Autodesk Inventor part; units mm, degrees
ref_plane "Work Plane2" through (0, 5.93, 0) normal (0, 1, 0) x (1, 0, 0)
ref_plane "YZ Plane" through (0, 0, 0) normal (1, 0, 0) x (0, 1, 0)
ref_plane "XZ Plane" through (0, 0, 0) normal (0, 1, 0) x (-1, 0, 0)
ref_plane "Work Plane2" through (0, 5.93, 0) normal (0, 1, 0) x (1, 0, 0)
sketch "Sketch7" plane through (0, 5.93, 0) normal (0, 1, 0) x (1, 0, 0)
  line L0 (-68.89, 72.25) -> (-68.89, 75.38)
  line L1 (-70.59, 75.38) -> (-68.89, 75.38)
  line L2 (-70.59, 83.0068) -> (-70.59, 75.38)
  line L3 (-64.9127, 88.12) -> (-70.59, 83.0068)
  line L4 (-5, 88.12) -> (-64.9127, 88.12)
  arc A0 (1.7, 81.42) -> (-5, 88.12) centre (-5, 81.42) ccw
  line L5 (1.7, 5) -> (1.7, 81.42)
  arc A1 (-5, -1.7) -> (1.7, 5) centre (-5, 5) ccw
  line L6 (-64.9127, -1.7) -> (-5, -1.7)
  line L7 (-70.59, 3.4132) -> (-64.9127, -1.7)
  line L8 (-70.59, 14.5) -> (-70.59, 3.4132)
  line L9 (-68.89, 14.5) -> (-70.59, 14.5)
  line L10 (-68.89, 14.5) -> (-68.89, 17.63)
  line L11 (-70.59, 17.63) -> (-68.89, 17.63)
  line L12 (-70.59, 47.6) -> (-70.59, 17.63)
  line L13 (-68.89, 47.6) -> (-70.59, 47.6)
  line L14 (-68.89, 47.6) -> (-68.89, 50.73)
  line L15 (-70.59, 50.73) -> (-68.89, 50.73)
  line L16 (-70.59, 72.25) -> (-70.59, 50.73)
  line L17 (-68.89, 72.25) -> (-70.59, 72.25)
  line L18 (5.3534, 92.34) -> (10.14, 87.0271)
  line L19 (-69.6869, 92.34) -> (5.3534, 92.34)
  line L20 (-73.78, 86.0365) -> (-69.6869, 92.34)
  line L21 (-73.78, 75.38) -> (-73.78, 86.0365)
  line L22 (-73.78, 75.38) -> (-73.78, 72.25)
  line L23 (-73.78, 50.73) -> (-73.78, 72.25)
  line L24 (-73.78, 50.73) -> (-73.78, 47.6)
  line L25 (-73.78, 17.63) -> (-73.78, 47.6)
  line L26 (-73.78, 17.63) -> (-73.78, 14.5)
  line L27 (-73.78, -2.6865) -> (-73.78, 14.5)
  line L28 (-69.6869, -8.99) -> (-73.78, -2.6865)
  line L29 (4.8271, -8.99) -> (-69.6869, -8.99)
  line L30 (10.14, -4.2034) -> (4.8271, -8.99)
  line L31 (10.14, 87.0271) -> (10.14, -4.2034)
  line L32 (-5, 0) -> (-64.26, 0)
  line L33 (-68.89, 4.17) -> (-64.26, 0)
  line L34 (-68.89, 4.17) -> (-68.89, 14.5)
  line L35 (-68.89, 17.63) -> (-68.89, 47.6)
  line L36 (-68.89, 50.73) -> (-68.89, 72.25)
  line L37 (-68.89, 75.38) -> (-68.89, 82.25)
  line L38 (-64.26, 86.42) -> (-68.89, 82.25)
  line L39 (-64.26, 86.42) -> (-5, 86.42)
  arc A2 (0, 81.42) -> (-5, 86.42) centre (-5, 81.42) ccw
  line L40 (0, 81.42) -> (0, 5)
  arc A3 (-5, 0) -> (0, 5) centre (-5, 5) ccw
  line L41 (-68.89, 14.5) -> (-70.59, 14.5)
  line L42 (-68.89, 14.5) -> (-68.89, 75.38)
  point P0 (0, 0)
extrude "Extrusion6" add sketch "Sketch7" along normal blind 5 contours L0 L37 L38 L39 A2 L40 A3 L32 L33 L34 L10 L35 L14 L36
sketch "Sketch8" plane through (0, 10.93, 0) normal (0, 1, 0) x (1, 0, 0)
  line L0 (-64.26, 0) -> (-64.26, 16.2)
  line L1 (-64.26, 16.2) -> (-64.26, 17.765)
  line L2 (-64.26, 17.765) -> (-41.26, 17.765)
  line L3 (-64.26, 17.765) -> (-64.26, 15.765)
  line L4 (-64.26, 15.765) -> (-41.26, 15.765)
  line L5 (-41.26, 15.765) -> (-41.26, 3.765)
  line L6 (-41.26, 3.765) -> (-64.26, 3.765)
  line L7 (-64.26, 3.765) -> (-64.26, 15.765)
  line L8 (-64.26, 9.765) -> (-66.573, 9.765)
  circle A0 centre (-66.573, 9.765) radius 1
  line L9 (-41.26, 9.765) -> (-38.947, 9.765)
  circle A1 centre (-38.947, 9.765) radius 1
  line L10 (-64.26, 17.765) -> (-64.26, 19.765)
  line L11 (-64.26, 19.765) -> (-41.26, 19.765)
  line L12 (-41.26, 19.765) -> (-41.26, 31.765)
  line L13 (-41.26, 31.765) -> (-64.26, 31.765)
  line L14 (-64.26, 31.765) -> (-64.26, 19.765)
  line L15 (-64.26, 25.765) -> (-66.573, 25.765)
  circle A2 centre (-66.573, 25.765) radius 1
  line L16 (-41.26, 25.765) -> (-38.947, 25.765)
  circle A3 centre (-38.947, 25.765) radius 1
  point P0 (0, 0)
  dimension "d56" = 16.2
  dimension "d57" = 1.565
  dimension "d58" = 23
  dimension "d59" = 90
  dimension "d60" = 2
  dimension "d61" = 23
  dimension "d62" = 12
  dimension "d63" = 2.313
  dimension "d64" = 2
  dimension "d65" = 2.313
  dimension "d66" = 2
  dimension "d67" = 2
  dimension "d68" = 23
  dimension "d69" = 12
  dimension "d70" = 2.313
  dimension "d71" = 2
  dimension "d73" = 2
extrude "Extrusion7" cut sketch "Sketch8" against normal up to surface (5 mm away)
sketch "Sketch9" plane through (0, 10.93, 0) normal (0, 1, 0) x (1, 0, 0)
  line L0 (-5, 86.42) -> (-64.26, 86.42)
  line L1 (-64.26, 86.42) -> (-64.26, 75.38)
  line L2 (-64.26, 75.38) -> (-64.26, 73.815)
  line L3 (-64.26, 73.815) -> (-64.26, 79.815)
  line L4 (-64.26, 79.815) -> (-41.26, 79.815)
  line L5 (-64.26, 73.815) -> (-66.39, 73.815)
  circle A0 centre (-66.39, 73.815) radius 1
  line L6 (-41.26, 79.815) -> (-41.26, 67.815)
  line L7 (-41.26, 67.815) -> (-64.26, 67.815)
  line L8 (-64.26, 67.815) -> (-64.26, 73.815)
  line L9 (-41.26, 73.815) -> (-39.13, 73.815)
  circle A1 centre (-39.13, 73.815) radius 1
  point P0 (0, 0)
  dimension "d76" = 11.04
  dimension "d77" = 1.565
  dimension "d79" = 6
  dimension "d80" = 23
  dimension "d82" = 2.13
  dimension "d85" = 2
  dimension "d88" = 12
  dimension "d89" = 23
  dimension "d90" = 2.13
  dimension "d91" = 2
extrude "Extrusion8" cut sketch "Sketch9" against normal up to surface (5 mm away)
sketch "Sketch10" plane through (0, 10.93, 0) normal (0, 1, 0) x (1, 0, 0)
  arc A0 (0, 81.42) -> (-5, 86.42) centre (-5, 81.42) ccw
  line L0 (0, 81.42) -> (0, 49.165)
  line L1 (0, 49.165) -> (-5, 49.165)
  line L2 (-5, 49.165) -> (-5, 51.165)
  line L3 (-5, 49.165) -> (-5, 47.165)
  line L4 (-5, 51.165) -> (-28, 51.165)
  line L5 (-28, 51.165) -> (-28, 63.165)
  line L6 (-28, 63.165) -> (-5, 63.165)
  line L7 (-5, 63.165) -> (-5, 51.165)
  line L8 (-5, 47.165) -> (-28, 47.165)
  line L9 (-28, 47.165) -> (-28, 35.165)
  line L10 (-28, 35.165) -> (-5, 35.165)
  line L11 (-5, 35.165) -> (-5, 47.165)
  line L12 (-28, 41.165) -> (-30.13, 41.165)
  line L13 (-5, 41.165) -> (-2.87, 41.165)
  circle A1 centre (-30.13, 41.165) radius 1
  circle A2 centre (-2.87, 41.165) radius 1
  line L14 (-28, 57.165) -> (-30.13, 57.165)
  line L15 (-5, 57.165) -> (-2.87, 57.165)
  circle A3 centre (-30.13, 57.165) radius 1
  circle A4 centre (-2.87, 57.165) radius 1
  point P0 (0, 0)
  dimension "d92" = 32.255
  dimension "d93" = 5
  dimension "d94" = 2
  dimension "d95" = 2
  dimension "d96" = 23
  dimension "d97" = 12
  dimension "d98" = 23
  dimension "d99" = 12
  dimension "d100" = 2.13
  dimension "d101" = 2.13
  dimension "d102" = 2
  dimension "d103" = 2
  dimension "d104" = 2.13
  dimension "d105" = 2.13
  dimension "d106" = 2
  dimension "d107" = 2
extrude "Extrusion9" cut sketch "Sketch10" against normal up to surface (5 mm away)
properties part number "Robotic Hand Tray"
Here's how the part is built. I have some questions about the finished solid (model axes, mm). A direction names the side the tool comes from. Round coordinates to 2 decimals unless told otherwise and drop trailing zeros. Write each loop counter-clockwise with the first axis right and the second up, starting at its lowest first coordinate (ties: lowest second). Pieces come first, ordered by that corner, then holes. Notation, with made-up numbers: (81, -0.75) -> (140, -0.75) arc R36 cw to (140, 36.25) -> close; hole circle Ø7 at (1.5, -13). An arc over 180 degrees is marked (long way). One line per item, written item: value.
1) Suppose I cut it at C-C on x = -30.13. List the corners of the cut face in (y, z) for me (3 decimals).
Filled sheet:
outline: (5.93, -86.42) -> (10.93, -86.42) -> (10.93, -58.165) -> (5.93, -58.165) -> close; (5.93, -56.165) -> (10.93, -56.165) -> (10.93, -42.165) -> (5.93, -42.165) -> close; (5.93, -40.165) -> (10.93, -40.165) -> (10.93, 0) -> (5.93, 0) -> close
2) Suppose I cut it at D-D on y = 7.85. Give the number of separate pieces and of enclosed holes in the cut face, plus the area to 3 significant figures.
Filled sheet:
separate pieces: 1
enclosed holes: 15
area: 4,510 mm2
3) Suppose I cut it at B-B on z = -36.5. List the corners of the cut face in (x, y) for me.
Filled sheet:
outline: (-68.89, 5.93) -> (-28, 5.93) -> (-28, 10.93) -> (-68.89, 10.93) -> close; (-5, 5.93) -> (0, 5.93) -> (0, 10.93) -> (-5, 10.93) -> close
4) For faces 3 (the face through (-68.89, 8, -43)), 4 (the face through (-53, 8, -31.765)), which set-ups out of +Z, -Z, +X, -X, +Y, -Y let a thin tool reach every point of the face, with its end or its side?
Filled sheet:
face 3: +Z, -Z, -X, +Y, -Y
face 4: +Y, -Y
5) If I drill on line 1 (Z direction, x = -15.5, y = 6.85) (3 decimals); line 2 (X direction, y = 6.9, z = -57); line 3 (Z direction, x = -64, y = 8.2) (3 decimals), over which ranges is the centre line in solid material (lowest first)? Write a range as [from, to].
Filled sheet:
line 1: z = [-86.42, -63.165], [-51.165, -47.165], [-35.165, 0]
line 2: x = [-68.89, -31.12], [-29.14, -28], [-5, -3.86], [-1.88, 0]
line 3: z = [-86.42, -79.815], [-67.815, -31.765], [-19.765, -15.765], [-3.765, 0]
6) We'd pull the mould along X, two halves only. Please class faces 1 (the face through (-39.684, 8.465, -26.441)), 2 (the face through (-66.5, 8.4, -84.4)): released by +X, released by -X, zero draft, split by the parting line, or undercut.
Filled sheet:
face 1: undercut
face 2: released by -X
7) I'm going to push a flat-ended pin straight in: pin 1 Ø1.6 at (x, z) = (-38.947, -9.765) entering from +Y. Where does the tip first touch, or does it pass through?
Filled sheet:
pin 1: passes through
8) Suppose I cut it at A-A on x = -49. List the corners of the cut face in (y, z) for me (3 decimals), plus the area to 3 significant figures.
Filled sheet:
outline: (5.93, -86.42) -> (10.93, -86.42) -> (10.93, -79.815) -> (5.93, -79.815) -> close; (5.93, -67.815) -> (10.93, -67.815) -> (10.93, -31.765) -> (5.93, -31.765) -> close; (5.93, -19.765) -> (10.93, -19.765) -> (10.93, -15.765) -> (5.93, -15.765) -> close; (5.93, -3.765) -> (10.93, -3.765) -> (10.93, 0) -> (5.93, 0) -> close
area: 252 mm2
